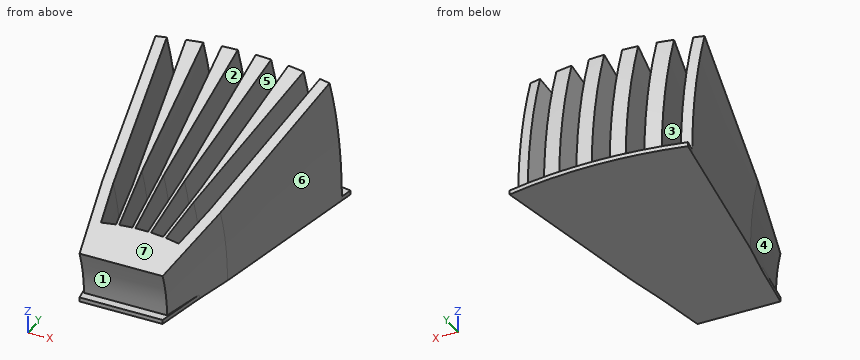
from build123d import *

# Parameters (mm, degrees)
REVOLUTION_ANGLE = 20
PAD_DEPTH        = 2


with BuildPart() as part:
    # Sketch → Revolution (revolve)
    with BuildSketch(Plane.XY):
        Polygon((-18.372564, 87.184066), (-22.823988, 108.307586), (-36.154546, 187.797393), (-41.085685, 186.970434), (-27.854335, 108.072199), (-19.606168, 68.93184), (19.606168, 68.93184), (27.854335, 108.072199), (41.085685, 186.970434), (36.154546, 187.797393), (22.823988, 108.307586), (18.372564, 87.184066), (11.764837, 88.292191), (14.448033, 109.712246), (27.778591, 189.202053), (20.095372, 190.164496), (14.105719, 118.233415), (10.376892, 88.466053), (4.397586, 88.963946), (5.643392, 118.938068), (11.633046, 190.869148), (4.245807, 191.176182), (4.245807, 118.996155), (3, 89.022034), (-3, 89.022034), (-4.245807, 118.996155), (-4.245807, 191.176182), (-11.633046, 190.869148), (-5.643392, 118.938068), (-4.397586, 88.963946), (-10.376892, 88.466053), (-14.105719, 118.233415), (-20.095372, 190.164496), (-27.778591, 189.202053), (-14.448033, 109.712246), (-11.764837, 88.292191), align=None)
    revolve(axis=Axis((0, 0, 0), (1, 0, 0)), revolution_arc=REVOLUTION_ANGLE)

    # Sketch001 → Pad (new body)
    with BuildSketch(Plane.XY):
        with BuildLine():
            ThreePointArc((42.112464, 192.811715), (0, 197.35708), (-42.112464, 192.811715))
            Line((-42.112464, 192.811715), (-19.606168, 64.774741))
            Line((-19.606168, 64.774741), (19.606168, 64.774741))
            Line((19.606168, 64.774741), (42.112464, 192.811715))
        make_face()
    extrude(amount=PAD_DEPTH)


solid = part.part
Geometry: final body of the model. Coordinates: model frame, mm. Face numbers are marked on the shaded views. A direction names the side the tool comes from. Round coordinates to 2 decimals unless told otherwise and drop trailing zeros. Order: outer loops, then holes, each group sorted by start corner. A loop starts at its lowest first (then second) coordinate and runs counter-clockwise, first axis right, second up.
Q1. Material intervals for probe 1 along X at (y, z) = (119, 21.5); probe 2 along X at (y, z) = (160, 34); probe 3 along Z at (x, y) = (-9, 108.5), sorted ascending.
Result sheet:
probe 1: x = -30.01 to -24.94, -16.33 to -14.33, -5.81 to -4.25, 4.25 to 5.81, 14.33 to 16.33, 24.94 to 30.01
probe 2: x = -37.16 to -32.09, -23.48 to -17.88, -9.36 to -4.25, 4.25 to 9.36, 17.88 to 23.48, 32.09 to 37.16
probe 3: z = 0 to 2
Q2. Access query for the marked faces 1, 2, 3 and 4. Directions: +Z, -Z, +X, -X, +Y, -Y. A direction counts if a zero-diameter tool reaches every point of the face in a straight line with its end or side. Return the directions, or none.
Result sheet:
face 1: +X, -X, -Y
face 2: +Z, +Y
face 3: none
face 4: -X, -Y
Q3. Section B-B, the plane x = 9. Output: boundary loops of the cut face in (y, z), and give its area (3 significant figures).
Result sheet:
outline: (64.77, 0) - (197.15, 0) - (197.15, 2) - (190.97, 2) arc R190.98 ccw to (179.46, 65.32) - (149.64, 54.47) arc R159.25 cw to (159.24, 2) - (88.56, 2) arc R88.58 ccw to (83.24, 30.3) - (64.77, 23.58) arc R68.93 cw to (68.9, 2) - (64.77, 2) - close
area: 2,640 mm2
Q4. Section A-A, the plane z = 59.5. Give the number of separate pieces and of enclosed holes in the cut face, and give its area (3 significant figures).
Result sheet:
separate pieces: 6
enclosed holes: 0
area: 623 mm2
Q5. Mould query, pull axis X, two halves, no side actions, for the marked faces 5, 6 and 7. Classes: released by +X, released by -X, zero draft, split by the parting line, or undercut.
Result sheet:
face 5: undercut
face 6: released by +X
face 7: zero draft
Q6. Section D-D, the plane x = 32. Output: boundary loops of the cut face in (y, z).
Result sheet:
outline: (124.78, 45.42) arc R132.79 cw to (132.79, 0) - (194.75, 0) - (194.75, 2) - (163.01, 2) arc R163.02 ccw to (153.19, 55.76) - close
Q7. Pin query (flat end, axial travel): pin 1 (12 mm diameter, centred on y = 144, z = 25.5, fed in from +X); pin 2 (10 mm diameter, centred on x = -10, z = 16, fed in from -Y); pin 3 (20 mm diameter, centred on x = 1.5, y = 77.5, fed in from +Z); pin 4 (1.5 mm diameter, centred on x = 17, y = 115.5, fed in from -Z). Return the tip coordinate at first contact, or that it passes through.
Result sheet:
pin 1: stops at x = 35.26
pin 2: stops at y = 65.66
pin 3: stops at z = 31.8
pin 4: stops at z = 0
